Autodesk Inventor part; units mm, degrees
ref_plane "YZ Plane" through (0, 0, 0) normal (1, 0, 0) x (0, 1, 0)
ref_plane "XZ Plane" through (0, 0, 0) normal (0, 1, 0) x (-1, 0, 0)
ref_plane "XY Plane" through (0, 0, 0) normal (0, 0, 1) x (1, 0, 0)
sketch "草图1" plane through (0, 0, 0) normal (0, 1, 0) x (-1, 0, 0)
  line L0 (0, 0) -> (50, 0)
  line L1 (50, 0) -> (50, -20)
  line L2 (50, -20) -> (0, -20)
  line L3 (0, -20) -> (0, 0)
  line L4 (35, -20) -> (15, -20)
  line L5 (15, -20) -> (15, -70)
  line L6 (15, -70) -> (35, -70)
  line L7 (35, -70) -> (35, -20)
  line L8 (25, 0) -> (25, -7.1636)
  line L9 (50, -20) -> (35, -70)
  line L10 (15, -70) -> (0, -20)
  circle A0 centre (40, -10) radius 2.55
  circle A1 centre (10, -10) radius 2.55
  circle A2 centre (25, -30) radius 2.55
  circle A3 centre (25, -60) radius 2.55
  line L11 (50, -10) -> (45.4992, -10)
  dimension "d0" = 50
  dimension "d1" = 20
  dimension "d2" = 20
  dimension "d3" = 50
  dimension "d4" = 5.1
  dimension "d5" = 10
  dimension "d6" = 10
  dimension "d7" = 10
extrude "拉伸1" add sketch "草图1" along normal blind 3
chamfer "倒角1" distance 4 angle 45 2 edges at (0, 1.5, 0) (-50, 1.5, 0)
chamfer "倒角2" distance 4 angle 45 2 edges at (-15, 1.5, -70) (-35, 1.5, -70)
sketch "草图2" plane through (0, 3, 0) normal (0, 1, 0) x (1, 0, 0)
  line L0 (-50, 20) -> (-50, 4)
  line L1 (-50, 4) -> (0, 4)
  line L2 (0, 4) -> (0, -20)
  line L3 (0, -20) -> (-50, -20)
  line L4 (-50, -20) -> (-50, 4)
  line L5 (0, 4) -> (0, 20)
  line L6 (-46, 0) -> (-4, 0)
  circle A0 centre (-40, -10) radius 2.5
  circle A1 centre (-10, -10) radius 2.5
  circle A2 centre (-40, 10) radius 2.55
  line L7 (-40, 10) -> (-10, 10)
  line L8 (-10, 10) -> (-10, -10)
  line L9 (-10, -10) -> (-40, -10)
  line L10 (-40, -10) -> (-40, 10)
  circle A3 centre (-10, 10) radius 2.55
  point P0 (0, 0)
  point P1 (-40, 0)
  point P2 (-40, 4)
  point P3 (-10, 4)
  point P4 (-10, 0)
  dimension "d16" = 20
  dimension "d17" = 4
  dimension "d18" = 5
  dimension "d19" = 5
  dimension "d20" = 10
extrude "拉伸2" add sketch "草图2" against normal up to surface (3 mm away) contours L1 L10 A0 L9 A1 L8 L2 L3 L4 | L6 L8 A1 L9 A0 L10
chamfer "倒角3" distance 4 angle 45 2 edges at (-50, 1.5, 20) (0, 1.5, 20)
properties part number "body_fix2_camera"
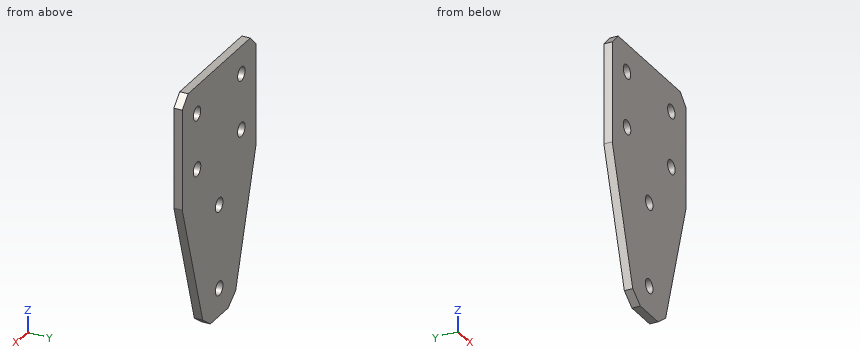
Can you work these out from the model? Positions are in its coordinate system, mm. Coordinates: 2 decimals unless noted, no trailing zeros. Write each loop counter-clockwise with the first axis right and the second up, starting at its lowest first coordinate (ties: lowest second). Pieces come first, ordered by that corner, then holes. Notation, with made-up numbers: (-4.75, 53.25) - (13.25, 53.25) arc R12 ccw to (13.25, 57.25) - close; hole circle Ø9 at (19.25, 20). An arc over 180 degrees is marked (long way). Return JSON: item names as keys, results as strings. Group by question number.
Item 1: I'm going to push flat-ended pins straight in: pin 1 Ø1.5 at (y, z) = (1, -59) entering from +X (3 decimals); pin 2 Ø4.5 at (x, z) = (-25, -60) entering from +Y; pin 3 Ø1 at (y, z) = (0.5, -21) entering from +X. Where does each tip first touch, or does it pass through?
Item 2: If we section it at D-D (x = -25): Write out the boundary of the cut face in (y, z).
Item 3: If we section it at C-C (y = 1.2): Write out the boundary of the cut face in (x, z), then the cut area to 3 significant figures.
Item 4: If we section it at B-B (z = -30): Write out the boundary of the cut face in (x, y), then the cut area to 3 significant figures.
Item 5: If we section it at A-A (z = 10): Write out the boundary of the cut face in (x, y).
Item 6: Please list where these lines run through material, in increasing order: probe 1 along X at (y, z) = (1.5, 10); probe 2 along Z at (x, y) = (-25, 2.4); probe 3 along X at (y, z) = (0.2, -52.5).
Return value:
{
 "1": {"pin 1": "stops at x = -11.475", "pin 2": "passes through", "pin 3": "stops at x = -0.15"},
 "2": {"outline": "(0, -70) - (3, -70) - (3, -62.55) - (0, -62.55) - close; (0, -57.45) - (3, -57.45) - (3, -32.55) - (0, -32.55) - close; (0, -27.45) - (3, -27.45) - (3, 20) - (0, 20) - close"},
 "3": {"outline": "(-50, -20) - (-36.15, -66.17) - (-31, -70) - (-19, -70) - (-13.85, -66.17) - (0, -20) - (0, 16) - (-4, 20) - (-46, 20) - (-50, 16) - close; hole circle Ø5.1 at (-40, -10); hole circle Ø5 at (-40, 10); hole circle Ø5.1 at (-25, -60); hole circle Ø5.1 at (-25, -30); hole circle Ø5.1 at (-10, -10); hole circle Ø5 at (-10, 10)", "area": "3,600 mm^2"},
 "4": {"outline": "(-47, 0) - (-27.55, 0) - (-27.55, 3) - (-47, 3) - close; (-22.45, 0) - (-3, 0) - (-3, 3) - (-22.45, 3) - close", "area": "117 mm^2"},
 "5": {"outline": "(-50, 0) - (-42.5, 0) - (-42.5, 3) - (-50, 3) - close; (-37.5, 0) - (-12.5, 0) - (-12.5, 3) - (-37.5, 3) - close; (-7.5, 0) - (0, 0) - (0, 3) - (-7.5, 3) - close"},
 "6": {"probe 1": "x = -50 to -42.5, -37.5 to -12.5, -7.5 to 0", "probe 2": "z = -70 to -62.55, -57.45 to -32.55, -27.45 to 20", "probe 3": "x = -40.25 to -9.75"}
}
